Design review of the part built by this model. Coordinates are the model's own, in mm. Coordinates: 2 decimals unless noted, no trailing zeros. Loops run counter-clockwise (first coordinate to the right, second up) from the corner with the lowest first, then second, coordinate; pieces in that order, holes last. Notation, with made-up numbers: (-18, 59) -> (9, 59) arc R25 ccw to (9, 98) -> close; hole circle Ø2 at (6, 24.5). An arc over 180 degrees is marked (long way). Use a Markdown table: item, result. Add a question column.
Q1. For probe 1 along Y at (x, z) = (-15, 3); probe 2 along Y at (x, z) = (3.5, 5.5); probe 3 along Y at (x, z) = (165, 2.95), list the stretches that pass through material, from the lowest coordinate up.
Q2. Take a section at B-B on y = -17. Write out the cut boundary in (x, z), plus the area to 3 significant figures.
Q3. Take a section at C-C on x = 75. Write out the cut boundary in (y, z).
Q4. Take a section at D-D on y = 172.5. Write out the cut boundary in (x, z), plus the area to 3 significant figures.
Q5. Take a section at A-A on x = -15. Write out the cut boundary in (y, z).
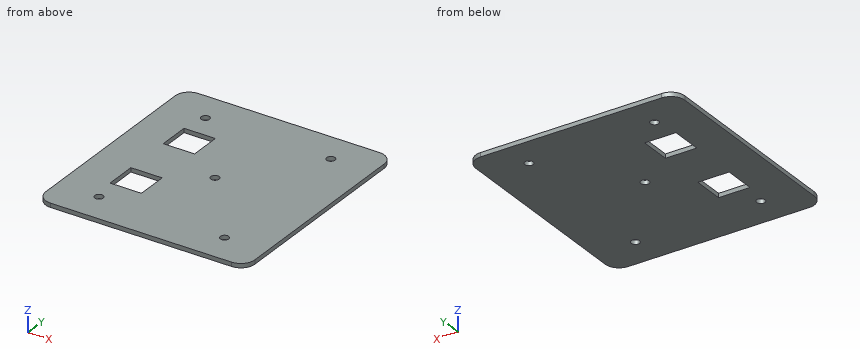
from build123d import *

# Parameters (mm, degrees)
SKETCH1_R           = 6
SKETCH1_W           = 45
SKETCH1_H           = 45
BOSS_EXTRUDE1_DEPTH = 6


with BuildPart() as part:
    # Sketch1 → Boss-Extrude1 (new body)
    with BuildSketch(Plane.XY):
        with BuildLine():
            Line((-55, -102.5), (205, -102.5))
            ThreePointArc((205, -102.5), (219.142135624, -96.642135624), (225, -82.5))
            Line((225, -82.5), (225, 197.5))
            ThreePointArc((225, 197.5), (219.142135624, 211.642135624), (205, 217.5))
            Line((205, 217.5), (-55, 217.5))
            ThreePointArc((-55, 217.5), (-69.142135624, 211.642135624), (-75, 197.5))
            Line((-75, 197.5), (-75, -82.5))
            ThreePointArc((-75, -82.5), (-69.142135624, -96.642135624), (-55, -102.5))
        make_face()
        with Locations((165, 172.5)):
            Circle(SKETCH1_R, mode=Mode.SUBTRACT)
        with Locations((-15, -57.5)):
            Circle(SKETCH1_R, mode=Mode.SUBTRACT)
        Polygon((22.5, -22.5), (-22.5, -22.5), (-22.5, 22.5), (0, 22.5), (22.5, 22.5), align=None, mode=Mode.SUBTRACT)
        with Locations((165, -57.5)):
            Circle(SKETCH1_R, mode=Mode.SUBTRACT)
        with Locations((0, 115)):
            Rectangle(SKETCH1_W, SKETCH1_H, mode=Mode.SUBTRACT)
        with Locations((-15, 172.5)):
            Circle(SKETCH1_R, mode=Mode.SUBTRACT)
        with Locations((75, 57.5)):
            Circle(SKETCH1_R, mode=Mode.SUBTRACT)
    extrude(amount=BOSS_EXTRUDE1_DEPTH)


solid = part.part
Answer list:
| question | item | result |
|---|---|---|
| 1 | probe 1 | -102.5 to -63.5, -51.5 to -22.5, 22.5 to 92.5, 137.5 to 166.5, 178.5 to 217.5 |
| 1 | probe 2 | -102.5 to -22.5, 22.5 to 92.5, 137.5 to 217.5 |
| 1 | probe 3 | -102.5 to -63.5, -51.5 to 166.5, 178.5 to 217.5 |
| 2 | outline | (-75, 0) -> (-22.5, 0) -> (-22.5, 6) -> (-75, 6) -> close; (22.5, 0) -> (225, 0) -> (225, 6) -> (22.5, 6) -> close |
| 2 | area | 1,530 mm² |
| 3 | outline | (-102.5, 0) -> (51.5, 0) -> (51.5, 6) -> (-102.5, 6) -> close; (63.5, 0) -> (217.5, 0) -> (217.5, 6) -> (63.5, 6) -> close |
| 4 | outline | (-75, 0) -> (-21, 0) -> (-21, 6) -> (-75, 6) -> close; (-9, 0) -> (159, 0) -> (159, 6) -> (-9, 6) -> close; (171, 0) -> (225, 0) -> (225, 6) -> (171, 6) -> close |
| 4 | area | 1,660 mm² |
| 5 | outline | (-102.5, 0) -> (-63.5, 0) -> (-63.5, 6) -> (-102.5, 6) -> close; (-51.5, 0) -> (-22.5, 0) -> (-22.5, 6) -> (-51.5, 6) -> close; (22.5, 0) -> (92.5, 0) -> (92.5, 6) -> (22.5, 6) -> close; (137.5, 0) -> (166.5, 0) -> (166.5, 6) -> (137.5, 6) -> close; (178.5, 0) -> (217.5, 0) -> (217.5, 6) -> (178.5, 6) -> close |
